Check sheet for the modelled part. Datum: model origin and axes. Units: mm. A direction names the side the tool comes from. Give positions to 0.01 mm unless a question says otherwise; leave off trailing zeros. Write each loop counter-clockwise with the first axis right and the second up, starting at its lowest first coordinate (ties: lowest second). Pieces come first, ordered by that corner, then holes. Notation, with made-up numbers: M 8,6 L 23,6 A18 cw 23,41 Z; hole C 75.5,-17 d3. An arc over 180 degrees is marked long. Use CSV: the item, a comma, the result in double quotes. Start each with the question number.
1. Cross-section at B-B, the plane z = -26. Enter the section's corners in (x, y).
2. Cross-section at C-C, the plane y = -11.5. Enter the section's corners in (x, z), and give its area (3 significant figures).
3. Depth check by flat-ended pin: P1, Ø10, axis at x = 20, z = -25.5, coming from the +Y side; P2, Ø1, axis at x = 34, z = -75.5, coming from the -Y side; P3, Ø1.5, axis at y = 5.5, z = -90, coming from the +X side. Enter the tip coordinate at first touch or a pass-through.
4. Scan lines: line 1 (X direction, y = -9, z = -76); line 2 (Y direction, x = 27, z = -24); line 3 (Z direction, x = 44.5, y = -1). Record each from-to range of solid material in increasing order.
5. Cross-section at D-D, the plane x = 60. Enter the section's corners in (y, z), and give its area (3 significant figures).
6. Mould release check, pull along Y, two halves, no side actions. Record for faces 6 (the face through (57, 1.27, -21)), 7 (the face through (25.044, 0.363, -4.357)), 8 (the face through (50.8, 0, -61)): +Y half, -Y half, draft (parallel to the pull), parting line (faces both ways), or undercut.
7. Cross-section at A-A, the plane x = 34. Enter the section's corners in (y, z).
8. Access from +Z, -Z, +X, -X, +Y, -Y to the whole of each face (thin tool, end or side, straight path). Record for faces 1 (the face through (57, 0, -37.16)), 2 (the face through (57, -1.27, -21)), 3 (the face through (25, -19.05, -73)), 4 (the face through (25, 19.05, -74)), 5 (the face through (25, 0, -124.525)).
from build123d import *

# Parameters (mm, degrees)
F1_DEPTH = 50.8
F3_DEPTH = 12.7


with BuildPart() as f1:
    # F0 (on Right) → F1 (new body)
    with BuildSketch(Plane.YZ):
        with BuildLine():
            ThreePointArc((25.4, 0), (0, -4.357951), (-25.4, 0))
            Line((-25.4, 0), (-25.4, -12.7))
            Line((-25.4, -12.7), (-19.05, -22.925066))
            Line((-19.05, -22.925066), (-19.05, -124.525066))
            Line((-19.05, -124.525066), (19.05, -124.525066))
            Line((19.05, -124.525066), (19.05, -22.925066))
            Line((19.05, -22.925066), (25.4, -12.7))
            Line((25.4, -12.7), (25.4, 0))
        make_face()
    extrude(amount=F1_DEPTH)

    # F2 (on face) → F3 (join)
    with BuildSketch(Plane.YZ.offset(50.8)):
        with BuildLine():
            ThreePointArc((1.27, -4.347367), (0, -4.357951), (-1.27, -4.347367))
            Line((-1.27, -4.347367), (-1.27, -37.160147))
            Line((-1.27, -37.160147), (1.27, -37.160147))
            Line((1.27, -37.160147), (1.27, -4.347367))
        make_face()
    extrude(amount=F3_DEPTH)


solid = f1.part
Worked answers:
1,outline,"M 0,-19.05 L 50.8,-19.05 L 50.8,-1.27 L 63.5,-1.27 L 63.5,1.27 L 50.8,1.27 L 50.8,19.05 L 0,19.05 Z"
2,outline,"M 0,-124.53 L 50.8,-124.53 L 50.8,-3.49 L 0,-3.49 Z"
2,area,"6,150 mm^2"
3,P1,"stops at y = 20.56"
3,P2,"stops at y = -19.05"
3,P3,"stops at x = 50.8"
4,line 1,"x = 0 to 50.8"
4,line 2,"y = -19.05 to 19.05"
4,line 3,"z = -124.53 to -4.35"
5,outline,"M -1.27,-37.16 L 1.27,-37.16 L 1.27,-4.35 A76.2 cw -1.27,-4.35 Z"
5,area,"83.3 mm^2"
6,face 6,"+Y half"
6,face 7,"undercut"
6,face 8,"draft"
7,outline,"M -25.4,-12.7 L -19.05,-22.93 L -19.05,-124.53 L 19.05,-124.53 L 19.05,-22.93 L 25.4,-12.7 L 25.4,0 A76.2 cw -25.4,0 Z"
8,face 1,"-Z, +X, +Y, -Y"
8,face 2,"+Z, -Z, +X, -Y"
8,face 3,"-Z, +X, -X, -Y"
8,face 4,"-Z, +X, -X, +Y"
8,face 5,"-Z, +X, -X, +Y, -Y"
